from build123d import *

# Parameters (mm, degrees)
SKETCH_1_W            = 300
SKETCH_1_H            = 300
EXTRUDE_1_DEPTH       = 1
EXTRUDE_2_OUTLINE_W   = 80
EXTRUDE_2_OUTLINE_H   = 40
EXTRUDE_2_OUTLINE_W_2 = 40
EXTRUDE_2_OUTLINE_H_2 = 80
EXTRUDE_2_DEPTH       = 1
SKETCH_3_R            = 3
CUT_EXTRUDE_6_DEPTH   = 359.144733033
SKETCH_4_R            = 2
CUT_EXTRUDE_7_DEPTH   = 359.144733033
SKETCH_5_R            = 1.5
SKETCH_5_R_2          = 11
CUT_EXTRUDE_8_DEPTH   = 359.144733033


# Read off the part's stored shape, not the designer's step: 凸台-拉伸2
with BuildPart() as part:
    # 草图1 → 凸台-拉伸1 (new body)
    with BuildSketch(Plane(origin=(0, 0, 0), x_dir=(1, 0, 0), z_dir=(0, 1, 0))):
        with Locations((91.102323194, -114.832625539)):
            Rectangle(SKETCH_1_W, SKETCH_1_H)
    extrude(amount=EXTRUDE_1_DEPTH)

    # 凸台-拉伸2 outline → 凸台-拉伸2 (cut)
    with BuildSketch(Plane(origin=(0, 0, 0), x_dir=(1, 0, 0), z_dir=(0, 1, 0))):
        with Locations((91.102323194, -14.832625539)):
            Rectangle(EXTRUDE_2_OUTLINE_W, EXTRUDE_2_OUTLINE_H)
        with Locations((91.102323194, -214.832625539)):
            Rectangle(EXTRUDE_2_OUTLINE_W, EXTRUDE_2_OUTLINE_H)
        with Locations((-8.897676806, -114.832625539)):
            Rectangle(EXTRUDE_2_OUTLINE_W_2, EXTRUDE_2_OUTLINE_H_2)
        with Locations((191.102323194, -114.832625539)):
            Rectangle(EXTRUDE_2_OUTLINE_W_2, EXTRUDE_2_OUTLINE_H_2)
    extrude(amount=EXTRUDE_2_DEPTH, mode=Mode.SUBTRACT)

    # 草图3 → 切除-拉伸6 (cut, through all)
    with BuildSketch(Plane(origin=(0, 0, 0), x_dir=(1, 0, 0), z_dir=(0, 1, 0))):
        with Locations(Location((-28.897676806, 5.167374461, 0), (0, 0, 270))):
            Circle(SKETCH_3_R)
        with Locations(Location((211.102323194, 5.167374461, 0), (0, 0, 270))):
            Circle(SKETCH_3_R)
        with Locations(Location((211.102323194, -229.359868174, 0), (0, 0, 270))):
            Circle(SKETCH_3_R)
        with Locations(Location((-28.897676806, -229.359868174, 0), (0, 0, 270))):
            Circle(SKETCH_3_R)
    extrude(amount=CUT_EXTRUDE_6_DEPTH, mode=Mode.SUBTRACT)

    # 草图4 → 切除-拉伸7 (cut, through all)
    with BuildSketch(Plane(origin=(0, 0, 0), x_dir=(1, 0, 0), z_dir=(0, 1, 0))):
        with Locations(Location((76.102323194, -184.832625539, 0), (0, 0, 270))):
            Circle(SKETCH_4_R)
        with Locations(Location((106.102323194, -184.832625539, 0), (0, 0, 270))):
            Circle(SKETCH_4_R)
        with Locations(Location((106.102323194, -174.832625539, 0), (0, 0, 270))):
            Circle(SKETCH_4_R)
        with Locations(Location((76.102323194, -174.832625539, 0), (0, 0, 270))):
            Circle(SKETCH_4_R)
        with Locations(Location((21.102323194, -99.832625539, 0), (0, 0, 270))):
            Circle(SKETCH_4_R)
        with Locations(Location((43.602323194, -99.832625539, 0), (0, 0, 270))):
            Circle(SKETCH_4_R)
        with Locations(Location((31.102323194, -128.332625539, 0), (0, 0, 270))):
            Circle(SKETCH_4_R)
        with Locations(Location((21.102323194, -128.332625539, 0), (0, 0, 270))):
            Circle(SKETCH_4_R)
        with Locations(Location((161.102323194, -99.832625539, 0), (0, 0, 270))):
            Circle(SKETCH_4_R)
        with Locations(Location((151.102323194, -99.832625539, 0), (0, 0, 270))):
            Circle(SKETCH_4_R)
        with Locations(Location((161.102323194, -129.832625539, 0), (0, 0, 270))):
            Circle(SKETCH_4_R)
        with Locations(Location((151.102323194, -129.832625539, 0), (0, 0, 270))):
            Circle(SKETCH_4_R)
        with Locations(Location((76.102323194, -44.832625539, 0), (0, 0, 270))):
            Circle(SKETCH_4_R)
        with Locations(Location((76.102323194, -54.832625539, 0), (0, 0, 270))):
            Circle(SKETCH_4_R)
        with Locations(Location((106.102323194, -54.832625539, 0), (0, 0, 270))):
            Circle(SKETCH_4_R)
        with Locations(Location((106.102323194, -44.832625539, 0), (0, 0, 270))):
            Circle(SKETCH_4_R)
    extrude(amount=CUT_EXTRUDE_7_DEPTH, mode=Mode.SUBTRACT)

    # 草图5 → 切除-拉伸8 (cut, through all)
    with BuildSketch(Plane(origin=(0, 0, 0), x_dir=(1, 0, 0), z_dir=(0, 1, 0))):
        with Locations(Location((150.102323194, -256.832625539, 0), (0, 0, 270))):
            Circle(SKETCH_5_R)
        with Locations(Location((181.102323194, -256.832625539, 0), (0, 0, 270))):
            Circle(SKETCH_5_R)
        with Locations(Location((150.102323194, -225.832625539, 0), (0, 0, 270))):
            Circle(SKETCH_5_R)
        with Locations(Location((181.102323194, -225.832625539, 0), (0, 0, 270))):
            Circle(SKETCH_5_R)
        with Locations(Location((1.102323194, -225.832625539, 0), (0, 0, 270))):
            Circle(SKETCH_5_R)
        with Locations(Location((32.102323194, -225.832625539, 0), (0, 0, 270))):
            Circle(SKETCH_5_R)
        with Locations(Location((32.102323194, -256.832625539, 0), (0, 0, 270))):
            Circle(SKETCH_5_R)
        with Locations(Location((1.102323194, -256.832625539, 0), (0, 0, 270))):
            Circle(SKETCH_5_R)
        with Locations(Location((16.602323194, -241.332625539, 0), (0, 0, 270))):
            Circle(SKETCH_5_R_2)
        with Locations(Location((165.602323194, -241.332625539, 0), (0, 0, 270))):
            Circle(SKETCH_5_R_2)
    extrude(amount=CUT_EXTRUDE_8_DEPTH, mode=Mode.SUBTRACT)


solid = part.part
Source: CAD feature listing. Evaluate the final solid. Frame: model axes, mm. Coordinates: 2 decimals unless noted, no trailing zeros. Loops run counter-clockwise (first coordinate to the right, second up) from the corner with the lowest first, then second, coordinate; pieces in that order, holes last. Notation, with made-up numbers: (-33.75, 80.25) -> (-13.75, 80.25) arc R32 cw to (-13.75, 106.25) -> close; hole circle Ø10 at (-12.75, 49.25). An arc over 180 degrees is marked (long way). Answer in a Markdown table with one row per item. Add a question column.
Q1. Section D-D on z = 241.5. Return the cut outline in (x, y).
Q2. Pull-direction query (X, two-part tool) for faces 1 (the face through (19.906, 0.493, 251.825)), 2 (the face through (89, 0, 113)); classes: pulls with the +X half, pulls with the -X half, needs draft (parallel to the pull), parting line crosses it, or undercut.
Q3. Section C-C on x = 99. Return the cut outline in (y, z).
Q4. Ray query, line 1 along Z through (x, y) = (115, 0.85); line 2 along X through (y, z) = (0.3, 111); line 3 along X through (y, z) = (0.85, 184.5). Return the intervals inside material, ascending.
Q5. Section B-B on z = 7. Return the cut outline in (x, y), and give its area (3 significant figures).
Q6. Section A-A on x = 189. Return the cut outline in (y, z).
Q7. Contact query for a flat-ended pin moving along its axis: pin 1 Ø3 at (x, z) = (151.1, 99.83) entering from +Y. Output: stop coordinate, or through.
Computed values:
| question | item | result |
|---|---|---|
| 1 | outline | (-58.9, 0) -> (5.6, 0) -> (5.6, 1) -> (-58.9, 1) -> close; (27.6, 0) -> (154.6, 0) -> (154.6, 1) -> (27.6, 1) -> close; (176.6, 0) -> (241.1, 0) -> (241.1, 1) -> (176.6, 1) -> close |
| 2 | face 1 | undercut |
| 2 | face 2 | needs draft |
| 3 | outline | (0, -35.17) -> (1, -35.17) -> (1, -5.17) -> (0, -5.17) -> close; (0, 34.83) -> (1, 34.83) -> (1, 194.83) -> (0, 194.83) -> close; (0, 234.83) -> (1, 234.83) -> (1, 264.83) -> (0, 264.83) -> close |
| 4 | line 1 | z = -35.17 to -5.17, 34.83 to 194.83, 234.83 to 264.83 |
| 4 | line 2 | x = -58.9 to -28.9, 11.1 to 171.1, 211.1 to 241.1 |
| 4 | line 3 | x = -58.9 to 74.13, 78.07 to 104.13, 108.07 to 241.1 |
| 5 | outline | (-58.9, 0) -> (51.1, 0) -> (51.1, 1) -> (-58.9, 1) -> close; (131.1, 0) -> (241.1, 0) -> (241.1, 1) -> (131.1, 1) -> close |
| 5 | area | 220 mm^2 |
| 6 | outline | (0, -35.17) -> (1, -35.17) -> (1, 74.83) -> (0, 74.83) -> close; (0, 154.83) -> (1, 154.83) -> (1, 264.83) -> (0, 264.83) -> close |
| 7 | pin 1 | passes through |
